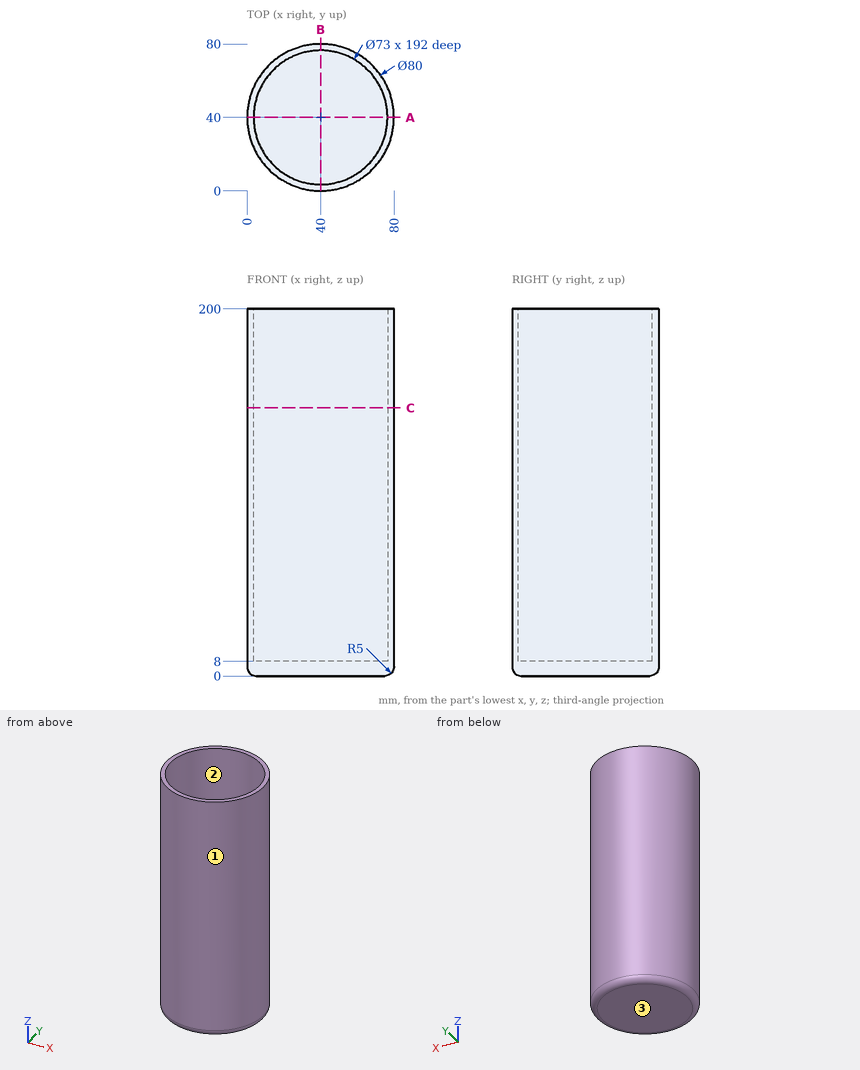
The figure shows three views and two pictorial views of one solid part (mm, origin at its lowest corner). Answer the questions. Give positions to 0.01 mm unless a question says otherwise; leave off trailing zeros. Order: outer loops, then holes, each group sorted by start corner. A loop starts at its lowest first (then second) coordinate and runs counter-clockwise, first axis right, second up. Notation, with made-up numbers: (-9.5, 16) -> (8.5, 16) arc R21 ccw to (8.5, 24) -> close; hole circle Ø5 at (53, 24). An arc over 180 degrees is marked (long way). One line per item, written item: value.
1) Find the intervals of material crossed by line 1 (Y direction, x = 40, z = 71); line 2 (Z direction, x = 54, y = 22); line 3 (X direction, y = 59, z = 82.5), in increasing order.
Reported:
line 1: y = 0 to 3.5, 76.5 to 80
line 2: z = 0 to 8
line 3: x = 4.8 to 8.84, 71.16 to 75.2
2) Flat-ended cylindrical pins translate along their axes: P1, Ø6, axis at x = 42.5, z = 128, coming from the +Y side; P2, Ø3, axis at x = 17.5, z = 172, coming from the +Y side; P3, Ø12, axis at x = 17, z = 92, coming from the -Y side. Find the tip coordinate at first contact, or state that the pin passes through.
Reported:
P1: stops at y = 80
P2: stops at y = 74.04
P3: stops at y = 3.79
3) Find section C-C, the plane z = 146. Determine the outline of the cut face in (x, y).
Reported:
outline: circle Ø80 at (40, 40); hole circle Ø73 at (40, 40)
4) Find section A-A, the plane y = 40. Determine the outline of the cut face in (x, z), plus the area to 3 significant figures.
Reported:
outline: (0, 5) arc R5 ccw to (5, 0) -> (75, 0) arc R5 ccw to (80, 5) -> (80, 200) -> (76.5, 200) -> (76.5, 8) -> (3.5, 8) -> (3.5, 200) -> (0, 200) -> close
area: 1,970 mm^2
5) Determine the mould class of the marked faces 1, 2 and 3 for opening direction Y: pulls with the +Y half, pulls with the -Y half, needs draft (parallel to the pull), parting line crosses it, or undercut.
Reported:
face 1: parting line crosses it
face 2: undercut
face 3: needs draft
